Geometry check sheet. Reference: the model listing, model coordinates, mm. Give positions to 0.01 mm unless a question says otherwise; leave off trailing zeros. Write each loop counter-clockwise with the first axis right and the second up, starting at its lowest first coordinate (ties: lowest second). Pieces come first, ordered by that corner, then holes.
(1) Cross-section at D-D (y = 1.7). Count the separate pieces of the cut face and the enclosed holes in it, and give its area (3 significant figures).
(2) Cross-section at A-A (z = -25.5). Record the boundary of the cut face in (x, y).
(3) Thickness scan on line 1 along X through (y, z) = (1.9, -51); line 2 along X through (y, z) = (0.25, 1); line 3 along X through (y, z) = (2.3, -10). Record the ranges inside material, lowest first.
(4) Cross-section at C-C (x = 127.5). Record the boundary of the cut face in (y, z), and give its area (3 significant figures).
(5) Depth check by flat-ended pin: P1, Ø1.5, axis at x = 24, y = 2, coming from the +Z side; P2, Ø1.5, axis at y = 1, z = 2, coming from the +X side; P3, Ø1.5, axis at y = 1, z = -41.5, coming from the +X side. Enter the tip coordinate at first touch or a pass-through.
(6) Cross-section at B-B (x = 76). Record the boundary of the cut face in (y, z), and give its area (3 significant figures).
```python
from build123d import *

# Parameters (mm, degrees)
EXTRUDE_1_DEPTH     = 3
FILLET_1_R          = 10
FILLET_2_R          = 10
SKETCH_2_W          = 11
SKETCH_2_H          = 28.4
SKETCH_2_W_2        = 15.55
SKETCH_2_H_2        = 40
CUT_EXTRUDE_1_DEPTH = 176.576963147
FILLET_3_R          = 4
EXTRUDE_START       = -3
EXTRUDE_2_DEPTH     = 3
FILLET_4_R          = 4


# Some blends are built 0.0001 mm under size
with BuildPart() as part:
    # 草图1 → 凸台-拉伸1 (new body)
    with BuildSketch(Plane(origin=(0, 0, 0), x_dir=(1, 0, 0), z_dir=(0, 1, 0))):
        Polygon((0, 0), (10, 0), (10, -3.5), (22, -3.5), (22, 0), (26.95, 0), (26.95, 3.4), (25.55, 3.4), (25.55, 6.8), (26.95, 6.8), (26.95, 10.3), (30.15, 10.3), (30.15, 6.8), (31.55, 6.8), (31.55, 3.4), (30.15, 3.4), (30.15, 0), (35.1, 0), (35.1, -3.5), (47.1, -3.5), (47.1, 0), (51.95, 0), (51.95, 3.4), (50.55, 3.4), (50.55, 6.8), (51.95, 6.8), (51.95, 10.3), (55.15, 10.3), (55.15, 6.8), (56.55, 6.8), (56.55, 3.4), (55.15, 3.4), (55.15, 0), (60.1, 0), (60.1, -3.5), (72.1, -3.5), (72.1, 0), (92.1, 0), (177.1, 50), (167.2, 50), (167.2, 53.5), (155.2, 53.5), (155.2, 50), (143.85, 50), (143.85, 46.5), (145.45, 46.5), (145.45, 43), (143.85, 43), (143.85, 39.6), (140.55, 39.6), (140.55, 43), (138.95, 43), (138.95, 46.5), (140.55, 46.5), (140.55, 50), (129.2, 50), (129.2, 53.5), (117.2, 53.5), (117.2, 50), (72.1, 50), (72.1, 53.5), (60.1, 53.5), (60.1, 50), (55.15, 50), (55.15, 46.6), (56.55, 46.6), (56.55, 43.2), (55.15, 43.2), (55.15, 39.7), (51.95, 39.7), (51.95, 43.2), (50.55, 43.2), (50.55, 46.6), (51.95, 46.6), (51.95, 50), (47.1, 50), (47.1, 53.5), (35.1, 53.5), (35.1, 50), (30.15, 50), (30.15, 46.6), (31.55, 46.6), (31.55, 43.2), (30.15, 43.2), (30.15, 39.7), (26.95, 39.7), (26.95, 43.2), (25.55, 43.2), (25.55, 46.6), (26.95, 46.6), (26.95, 50), (22, 50), (22, 53.5), (10, 53.5), (10, 50), (0, 50), align=None)
    extrude(amount=EXTRUDE_1_DEPTH)

    # 圆角1
    # the kernel refuses this fillet: 10 mm, written as the material it takes off along each edge
    with BuildSketch(Plane(origin=(177.1, -43.011578588, -50), x_dir=(-0.8619342151577696, 0, 0.5070201265633938), z_dir=(0, 1, 0))) as fillet_1_piece_1:
        with BuildLine():
            CenterArc((17.204631435, -10), FILLET_1_R, 90, 60.128922386)
            Line((8.53314873, -5.019499253), (8.359719076, -4.919889238))
            ThreePointArc((8.359719076, -4.919889238), (4.16517034, -2.68213647), (-0.101404025, -0.172386843))
            Line((-0.101404025, -0.172386843), (0, 0.2))
            Line((0, 0.2), (17.204631435, 0.2))
            Line((17.204631435, 0.2), (17.204631435, 0))
        make_face()
    extrude(amount=89.023157177, mode=Mode.SUBTRACT)

    # 圆角2
    fillet_2_edges = [part.edges().sort_by_distance(p)[0] for p in [
        (92.1, 1.5, 0),
        (0, 1.5, -50),
        (0, 1.5, 0),
    ]]
    fillet(fillet_2_edges, radius=FILLET_2_R - 0.0001)  # a hair under: the kernel refuses the full size

    # 草图2 → 切除-拉伸1 (cut, through all)
    with BuildSketch(Plane.XZ):
        Polygon((62.55, -6), (62.55, -44), (132.95, -44), (132.95, -30.990499855), (90.466150246, -6), align=None)
        with Locations((41.05, -25)):
            Rectangle(SKETCH_2_W, SKETCH_2_H)
        with Locations((12.775, -25)):
            Rectangle(SKETCH_2_W_2, SKETCH_2_H_2)
    extrude(amount=-CUT_EXTRUDE_1_DEPTH, mode=Mode.SUBTRACT)

    # 圆角3
    fillet_3_edges = [part.edges().sort_by_distance(p)[0] for p in [
        (62.55, 1.5, -6),
        (90.466150246, 1.5, -6),
        (132.95, 1.5, -30.990499855),
        (132.95, 1.5, -44),
        (62.55, 1.5, -44),
        (35.55, 1.5, -39.2),
        (35.55, 1.5, -10.8),
        (46.55, 1.5, -10.8),
        (46.55, 1.5, -39.2),
        (5, 1.5, -45),
        (5, 1.5, -5),
        (20.55, 1.5, -5),
        (20.55, 1.5, -45),
    ]]
    fillet(fillet_3_edges, radius=FILLET_3_R)

    # 草图3 → 凸台-拉伸2 (add)
    with BuildSketch(Plane.XZ.offset(EXTRUDE_START)):
        with BuildLine():
            Line((62.55, -40), (89.376917077, -6))
            ThreePointArc((89.376917077, -6), (90.427881528, -6.140534529), (91.404997583, -6.552263139))
            Line((91.404997583, -6.552263139), (66.55, -44))
            ThreePointArc((66.55, -44), (63.721572875, -42.828427125), (62.55, -40))
        make_face()
    extrude(amount=EXTRUDE_2_DEPTH)

    # 圆角4
    fillet_4_edges = [part.edges().sort_by_distance(p)[0] for p in [
        (91.404997583, 1.5, -6.552263139),
        (66.55, 1.5, -44),
        (89.376917077, 1.5, -6),
        (62.55, 1.5, -40),
    ]]
    fillet(fillet_4_edges, radius=FILLET_4_R)


solid = part.part
```
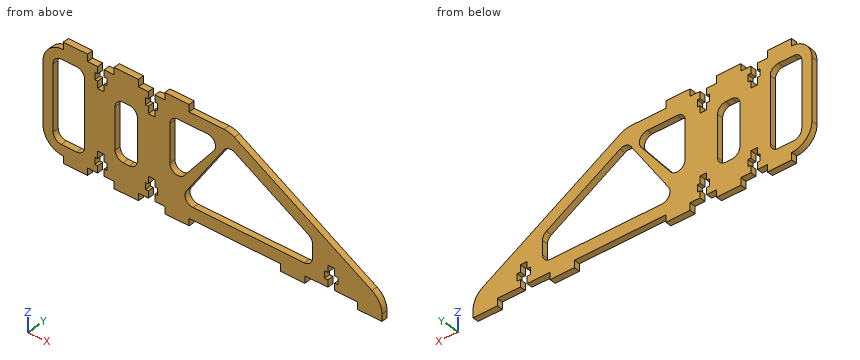
Reply:
1. separate pieces: 1
1. enclosed holes: 4
1. area: 3,960 mm2
2. outline: (0, 0) - (5, 0) - (5, 3) - (0, 3) - close; (20.55, 0) - (35.55, 0) - (35.55, 3) - (20.55, 3) - close; (46.55, 0) - (62.55, 0) - (62.55, 3) - (46.55, 3) - close; (73.99, 0) - (78.83, 0) - (78.83, 3) - (73.99, 3) - close; (123.62, 0) - (135.45, 0) - (135.45, 3) - (123.62, 3) - close
3. line 1: x = 10 to 22, 35.1 to 47.1, 60.1 to 72.1, 117.2 to 129.2, 155.2 to 167.2
3. line 2: x = 10 to 22, 35.1 to 47.1, 60.1 to 72.1
3. line 3: x = 0 to 5, 20.55 to 26.95, 30.15 to 51.95, 55.15 to 62.55, 85.13 to 89.12, 97.27 to 109.1
4. outline: (0, -53.5) - (3, -53.5) - (3, -44) - (0, -44) - close; (0, -27.78) - (3, -27.78) - (3, -20.82) - (0, -20.82) - close
4. area: 49.4 mm2
5. P1: stops at z = 0
5. P2: stops at x = 72.1
5. P3: stops at x = 163.65
6. outline: (0, -50) - (3, -50) - (3, -44) - (0, -44) - close; (0, -29.76) - (3, -29.76) - (3, -22.95) - (0, -22.95) - close; (0, -6) - (3, -6) - (3, 0) - (0, 0) - close
6. area: 56.4 mm2
